Check sheet for the modelled part. Datum: model origin and axes. Units: mm. Round coordinates to 2 decimals unless told otherwise and drop trailing zeros. Order: outer loops, then holes, each group sorted by start corner. A loop starts at its lowest first (then second) coordinate and runs counter-clockwise, first axis right, second up.
(1) Thickness scan on probe 1 along Y at (x, z) = (-12, 8.25); probe 2 along X at (y, z) = (2, 6.5); probe 3 along X at (y, z) = (-8.5, 11). Record the ranges inside material, lowest first.
(2) Mould release check, pull along Y, two halves, no side actions. Record for faces 1 (the cylindrical face through (50, 0, 4)), 2 (the cylindrical face through (-14.4, -1.8, 6.1)), 3 (the cylindrical face through (64.6, -1.8, 6.1)), 4 (the flat face through (-1, 16, 6)): released by +Y, released by -Y, zero draft, split by the parting line, or undercut.
(3) Sectioned sample at A-A, the plane y = 0. Enter the section's corners in (x, z).
(4) Sectioned sample at D-D, the plane x = 50. Enter the section's corners in (y, z), and give its area (3 significant figures).
(5) Sectioned sample at B-B, the plane x = -48. Enter the section's corners in (y, z), and give its area (3 significant figures).
(6) Sectioned sample at C-C, the plane z = 6. Enter the section's corners in (x, y), and give its area (3 significant figures).
```python
from build123d import *

# Parameters (mm, degrees)
IZIM1_W                     = 150
IZIM1_H                     = 32
Y_KSEKLIK_EKSTR_ZYON1_DEPTH = 12
IZIM2_R                     = 8
IZIM2_R_2                   = 9
KES_EKSTR_ZYON1_DEPTH       = 60
IZIM3_R                     = 3
KES_EKSTR_ZYON2_DEPTH       = 30


with BuildPart() as part:
    # Çizim1 → Yükseklik-Ekstrüzyon1 (new body)
    with BuildSketch(Plane.XY):
        Rectangle(IZIM1_W, IZIM1_H)
    extrude(amount=Y_KSEKLIK_EKSTR_ZYON1_DEPTH)

    # Çizim2 → Kes-Ekstrüzyon1 (cut)
    with BuildSketch(Plane(origin=(0, 16, 0), x_dir=(1, 0, 0), z_dir=(0, 1, 0))):
        with Locations((50, -12)):
            Circle(IZIM2_R)
        with Locations((-30, -12)):
            Circle(IZIM2_R_2)
    extrude(amount=-KES_EKSTR_ZYON1_DEPTH, mode=Mode.SUBTRACT)

    # Çizim3 → Kes-Ekstrüzyon2 (cut)
    with BuildSketch(Plane.XY.offset(12)):
        with Locations((67, 0)):
            Circle(IZIM3_R)
        with Locations((-48, 0)):
            Circle(IZIM3_R)
        with Locations((-12, 0)):
            Circle(IZIM3_R)
    extrude(amount=-KES_EKSTR_ZYON2_DEPTH, mode=Mode.SUBTRACT)


solid = part.part
```
Derived:
1. probe 1: y = -16 to -3, 3 to 16
1. probe 2: x = -75 to -50.24, -45.76 to -37.12, -22.88 to -14.24, -9.76 to 44.19, 55.81 to 64.76, 69.24 to 75
1. probe 3: x = -75 to -38.94, -21.06 to 42.06, 57.94 to 75
2. face 1: zero draft
2. face 2: undercut
2. face 3: undercut
2. face 4: released by +Y
3. outline: (-75, 0) - (-51, 0) - (-51, 12) - (-75, 12) - close; (-45, 0) - (-15, 0) - (-15, 12) - (-21, 12) arc R9 cw to (-39, 12) - (-45, 12) - close; (-9, 0) - (64, 0) - (64, 12) - (58, 12) arc R8 cw to (42, 12) - (-9, 12) - close; (70, 0) - (75, 0) - (75, 12) - (70, 12) - close
4. outline: (-16, 0) - (16, 0) - (16, 4) - (-16, 4) - close
4. area: 128 mm2
5. outline: (-16, 0) - (-3, 0) - (-3, 12) - (-16, 12) - close; (3, 0) - (16, 0) - (16, 12) - (3, 12) - close
5. area: 312 mm2
6. outline: (-75, -16) - (-36.71, -16) - (-36.71, 16) - (-75, 16) - close; (-23.29, -16) - (44.71, -16) - (44.71, 16) - (-23.29, 16) - close; (55.29, -16) - (75, -16) - (75, 16) - (55.29, 16) - close; hole circle Ø6 at (-48, 0); hole circle Ø6 at (-12, 0); hole circle Ø6 at (67, 0)
6. area: 3,950 mm2
